from build123d import *

# Parameters (mm, degrees)
BOSS_EXTRUDE1_DEPTH = 5.9
SKETCH2_R           = 2.475
CUT_EXTRUDE7_DEPTH  = 10.689525272


with BuildPart() as part:
    # Sketch1 → Boss-Extrude1 (new body)
    with BuildSketch(Plane.XY):
        Polygon((4.95, 0.3), (2.95, -1.7), (-2.95, -1.7), (-4.95, 0.3), (-4.95, 1.7), (-2.5, 1.7), (-2.5, 4.18), (2.5, 4.18), (2.5, 1.7), (4.95, 1.7), align=None)
    extrude(amount=BOSS_EXTRUDE1_DEPTH)

    # Sketch2 → Cut-Extrude7 (cut, through all)
    with BuildSketch(Plane(origin=(0, 4.18, 0), x_dir=(1, 0, 0), z_dir=(0, 1, 0))):
        with Locations(Location((0, -2.95, 0), (0, 0, 180))):
            Circle(SKETCH2_R)
    extrude(amount=-CUT_EXTRUDE7_DEPTH, mode=Mode.SUBTRACT)


solid = part.part
The listing builds one solid part. Answer for the finished solid, in the listing's coordinates (mm). A direction names the side the tool comes from. Round coordinates to 2 decimals unless told otherwise and drop trailing zeros. Order: outer loops, then holes, each group sorted by start corner. A loop starts at its lowest first (then second) coordinate and runs counter-clockwise, first axis right, second up. Notation, with made-up numbers: (-1.5, 65.25) - (31.5, 65.25) arc R26 cw to (31.5, 99.25) - close; hole circle Ø4 at (-28.75, 89). An arc over 180 degrees is marked (long way). Write item = value, one per line. Start each with the question number.
1) Section D-D, the plane z = 4.1 is taken. Write down the section's boundary in (x, y).
2) Section A-A, the plane z = 2.95 is taken. Write down the section's boundary in (x, y) (3 decimals).
3) Section C-C, the plane y = 0.85 is taken. Write down the section's boundary in (x, z) (3 decimals).
4) Given pin 1 (2.5 mm diameter, centred on y = 3, z = 4, fed in from -X), flat-ended and moving along its own axis, determine where the tip first touches the part or whether it passes through.
5) For faces 1 (the flat face through (-3.94, -0.71, 2.91)), 2 (the flat face through (-4, 1.7, 3)), 3 (the flat face through (4, 1.7, 3)), determine the directions among +Z, -Z, +X, -X, +Y, -Y from which every point of the face is accessible in a straight line to the end or side of a thin tool.
6) Section B-B, the plane x = 0 is taken. Write down the section's boundary in (y, z) (3 decimals).
7) Straight lines are drawn through the part: L1, parallel to Z at x = 0, y = 0.9 (3 decimals); L2, parallel to Z at x = -1.5, y = 3.15; L3, parallel to X at y = 2.15, z = 1.85. For each, find the intervals that lie inside material, in ascending order.
Results list:
q1.outline = (-4.95, 0.3) - (-2.95, -1.7) - (-2.19, -1.7) - (-2.19, 4.18) - (-2.5, 4.18) - (-2.5, 1.7) - (-4.95, 1.7) - close; (2.19, -1.7) - (2.95, -1.7) - (4.95, 0.3) - (4.95, 1.7) - (2.5, 1.7) - (2.5, 4.18) - (2.19, 4.18) - close
q2.outline = (-4.95, 0.3) - (-2.95, -1.7) - (-2.475, -1.7) - (-2.475, 4.18) - (-2.5, 4.18) - (-2.5, 1.7) - (-4.95, 1.7) - close; (2.475, -1.7) - (2.95, -1.7) - (4.95, 0.3) - (4.95, 1.7) - (2.5, 1.7) - (2.5, 4.18) - (2.475, 4.18) - close
q3.outline = (-4.95, 0) - (4.95, 0) - (4.95, 5.9) - (-4.95, 5.9) - close; hole circle Ø4.95 at (0, 2.95)
q4.pin_1 = -2.5
q5.face_1 = +Z, -Z, -X, -Y
q5.face_2 = +Z, -Z, -X, +Y
q5.face_3 = +Z, -Z, +X, +Y
q6.outline = (-1.7, 0) - (4.18, 0) - (4.18, 0.475) - (-1.7, 0.475) - close; (-1.7, 5.425) - (4.18, 5.425) - (4.18, 5.9) - (-1.7, 5.9) - close
q7.L1 = 0 to 0.475, 5.425 to 5.9
q7.L2 = 0 to 0.98, 4.92 to 5.9
q7.L3 = -2.5 to -2.22, 2.22 to 2.5
